Could you check a few things on this drawing? It's one solid part, dimensions in mm from its lowest x, y, z. A direction names the side the tool comes from. Coordinates: 2 decimals unless noted, no trailing zeros. Loops run counter-clockwise (first coordinate to the right, second up) from the corner with the lowest first, then second, coordinate; pieces in that order, holes last. Notation, with made-up numbers: M 50.5,36.25 L 108.5,36.25 A5 ccw 108.5,44.25 Z; hole C -34,9 d3. An arc over 180 degrees is marked long. Use one line per item in the form item = value. Start each with the question number.
(1) Please list where these lines run through material, in increasing order: L1, parallel to Y at x = 3, z = 17.75; L2, parallel to Z at x = 29.5, y = 3.5; L3, parallel to X at y = 9.25, z = 13.
(2) Imagine slicing it at C-C, the plane z = 17. Please give me the cut outline in (x, y), and give its area (3 significant figures).
(3) On a 3-axis mill with a long thin cutter (end or side, diameter ignored), from which of +Z, -Z, +X, -X, +Y, -Y can I reach the whole of each face in a straight line? I mean the marked faces 1, 2 and 3. Say none if no direction works.
(4) Imagine slicing it at D-D, the plane y = 1.75. Please give me the cut outline in (x, z).
(5) Will these pins go through, and if not, where does the flat tip stop? P1, Ø3, axis at x = 17.5, z = 2.5, coming from the -Y side; P2, Ø5, axis at x = 31, y = 17, coming from the +Z side; P3, Ø10, axis at y = 9.5, z = 9, coming from the +X side; P4, Ø4, axis at y = 6.5, z = 8, coming from the -X side.
(6) Imagine slicing it at A-A, the plane y = 4. Please give me the cut outline in (x, z).
(7) Imagine slicing it at B-B, the plane x = 31. Please give me the cut outline in (y, z).
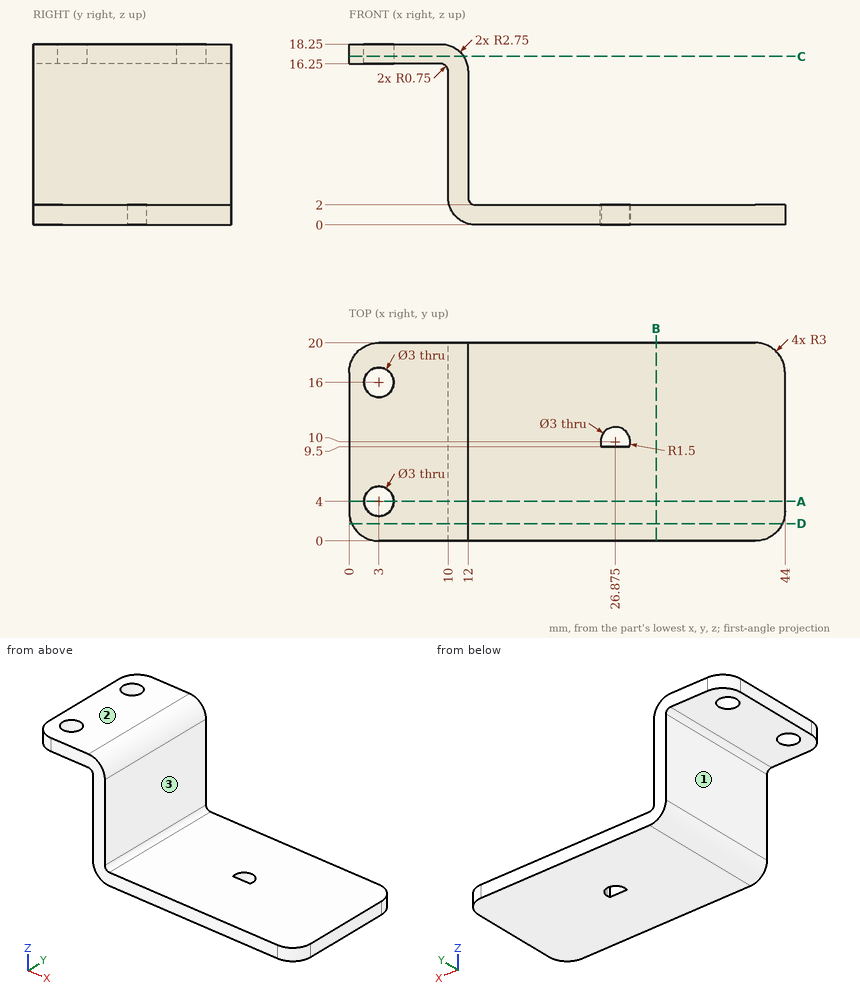
Answer:
q1.L1 = 0 to 2.5, 5.5 to 14.5, 17.5 to 20
q1.L2 = 0 to 2
q1.L3 = 10 to 12
q2.outline = M 0,3 A3 ccw 3,0 L 11.55,0 L 11.55,20 L 3,20 A3 ccw 0,17 Z; hole C 3,4 d3; hole C 3,16 d3
q2.area = 213 mm²
q3.face_1 = -Z, -X, +Y, -Y
q3.face_2 = +Z, +X, -X, +Y, -Y
q3.face_3 = +Z, +X, +Y, -Y
q4.outline = M 0.27,16.25 L 9.25,16.25 A0.75 cw 10,15.5 L 10,2.75 A2.75 ccw 12.75,0 L 43.73,0 L 43.73,2 L 12.75,2 A0.75 cw 12,2.75 L 12,15.5 A2.75 ccw 9.25,18.25 L 0.27,18.25 Z
q5.P1 = 0
q5.P2 = 2
q5.P3 = 12
q5.P4 = 10
q6.outline = M 0,16.25 L 1.5,16.25 L 1.5,18.25 L 0,18.25 Z; M 4.5,16.25 L 9.25,16.25 A0.75 cw 10,15.5 L 10,2.75 A2.75 ccw 12.75,0 L 44,0 L 44,2 L 12.75,2 A0.75 cw 12,2.75 L 12,15.5 A2.75 ccw 9.25,18.25 L 4.5,18.25 Z
q7.outline = M 0,0 L 20,0 L 20,2 L 0,2 Z
